```python
from build123d import *

# Parameters (mm, degrees)
SKETCH_1_R      = 2.5
SKETCH_1_R_2    = 3.5
SKETCH_1_R_3    = 3
EXTRUDE_1_DEPTH = 5
FILLET_1_R      = 20
FILLET_2_R      = 20
FILLET_3_R      = 50
FILLET_4_R      = 50
FILLET_5_R      = 50
FILLET_6_R      = 50
FILLET_7_R      = 50
FILLET_8_R      = 50


with BuildPart() as part:
    # 草图1 → 凸台-拉伸1 (new body)
    with BuildSketch(Plane(origin=(4.7625, 0, 0), x_dir=(0, 0, -1), z_dir=(1, 0, 0))):
        Polygon((-227, 0), (-227, -130), (-137, -195), (137, -195), (227, -130), (227, 0), (207, 130), (-207, 130), align=None)
        with Locations((-8, 85)):
            Circle(SKETCH_1_R, mode=Mode.SUBTRACT)
        with Locations((-8, 50)):
            Circle(SKETCH_1_R, mode=Mode.SUBTRACT)
        with Locations(Location((8, 50, 0), (0, 0, 180))):
            Circle(SKETCH_1_R, mode=Mode.SUBTRACT)
        with Locations(Location((8, 85, 0), (0, 0, 180))):
            Circle(SKETCH_1_R, mode=Mode.SUBTRACT)
        with Locations((-100, -175)):
            Circle(SKETCH_1_R_2, mode=Mode.SUBTRACT)
        with Locations((100, -175)):
            Circle(SKETCH_1_R_2, mode=Mode.SUBTRACT)
        with Locations(Location((167, 0, 0), (0, 0, 180))):
            Circle(SKETCH_1_R_2, mode=Mode.SUBTRACT)
        with Locations(Location((87, 0, 0), (0, 0, 180))):
            Circle(SKETCH_1_R_2, mode=Mode.SUBTRACT)
        with Locations(Location((-87, 0, 0), (0, 0, 180))):
            Circle(SKETCH_1_R_2, mode=Mode.SUBTRACT)
        with Locations(Location((-167, 0, 0), (0, 0, 180))):
            Circle(SKETCH_1_R_2, mode=Mode.SUBTRACT)
        with Locations(Location((-215, -50, 0), (0, 0, 180))):
            Circle(SKETCH_1_R_3, mode=Mode.SUBTRACT)
        Polygon((130, -155), (-130, -155), (-175, -120), (-115, -25), (115, -25), (175, -120), align=None, mode=Mode.SUBTRACT)
        Polygon((-144.568690861, -25), (-202, -25), (-202, -85), (-182.463427703, -85), align=None, mode=Mode.SUBTRACT)
        Polygon((182.463427703, -85), (144.568690861, -25), (202, -25), (202, -85), align=None, mode=Mode.SUBTRACT)
        Polygon((-185.552026081, 105), (-50, 105), (-50, 25), (-197.859718389, 25), align=None, mode=Mode.SUBTRACT)
        Polygon((50, 105), (50, 25), (197.859718389, 25), (185.552026081, 105), align=None, mode=Mode.SUBTRACT)
        with BuildLine():
            ThreePointArc((-215, -113.5), (-218, -110.5), (-215, -107.5))
            ThreePointArc((-215, -107.5), (-200.117904907, -105.540735012), (-186.25, -99.796460718))
            ThreePointArc((-186.25, -99.796460718), (-182.151923789, -100.894536929), (-183.25, -104.99261314))
            ThreePointArc((-183.25, -104.99261314), (-198.564990636, -111.336289969), (-215, -113.5))
        make_face(mode=Mode.SUBTRACT)
    extrude(amount=-EXTRUDE_1_DEPTH)

    # 圆角1
    fillet_1_edges = [part.edges().sort_by_distance(p)[0] for p in [
        (2.2625, 130, 207),
    ]]
    fillet(fillet_1_edges, radius=FILLET_1_R)

    # 圆角2
    fillet_2_edges = [part.edges().sort_by_distance(p)[0] for p in [
        (2.2625, 130, -207),
    ]]
    fillet(fillet_2_edges, radius=FILLET_2_R)

    # 圆角3
    fillet_3_edges = [part.edges().sort_by_distance(p)[0] for p in [
        (2.2625, 0, 227),
    ]]
    fillet(fillet_3_edges, radius=FILLET_3_R)

    # 圆角4
    fillet_4_edges = [part.edges().sort_by_distance(p)[0] for p in [
        (2.2625, 0, -227),
    ]]
    fillet(fillet_4_edges, radius=FILLET_4_R)

    # 圆角5
    fillet_5_edges = [part.edges().sort_by_distance(p)[0] for p in [
        (2.2625, -130, 227),
    ]]
    fillet(fillet_5_edges, radius=FILLET_5_R)

    # 圆角6
    fillet_6_edges = [part.edges().sort_by_distance(p)[0] for p in [
        (2.2625, -195, 137),
    ]]
    fillet(fillet_6_edges, radius=FILLET_6_R)

    # 圆角7
    fillet_7_edges = [part.edges().sort_by_distance(p)[0] for p in [
        (2.2625, -195, -137),
    ]]
    fillet(fillet_7_edges, radius=FILLET_7_R)

    # 圆角8
    fillet_8_edges = [part.edges().sort_by_distance(p)[0] for p in [
        (2.2625, -130, -227),
    ]]
    fillet(fillet_8_edges, radius=FILLET_8_R)


solid = part.part
```
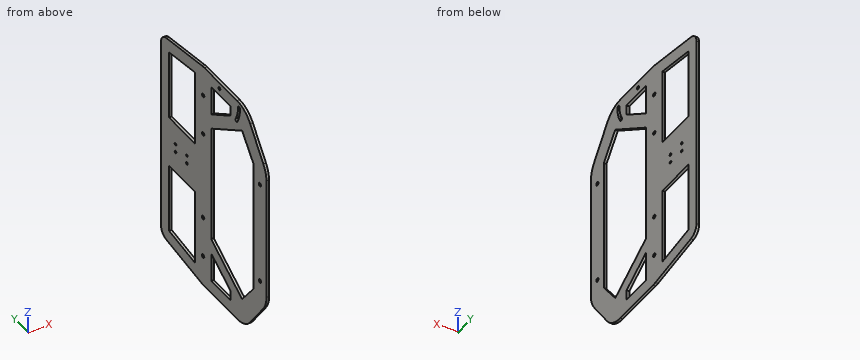
Here's how the part is built. I have some questions about the finished solid (model axes, mm). Coordinates: 2 decimals unless noted, no trailing zeros. Loops run counter-clockwise (first coordinate to the right, second up) from the corner with the lowest first, then second, coordinate; pieces in that order, holes last. Notation, with made-up numbers: M 0.5,6.25 L 43.5,6.25 A28 cw 43.5,41.25 Z; hole C -29,84.25 d8. An arc over 180 degrees is marked long. One line per item, written item: value.
1. Imagine slicing it at D-D (x = 2). State how many separate pieces and enclosed holes the cut face has, and give its area (3 significant figures).
Geometry says:
separate pieces: 1
enclosed holes: 17
area: 72,700 mm2
2. Please list where these lines run through material, in increasing order: probe 1 along Y at (x, z) = (2.65, 8.5); probe 2 along Y at (x, z) = (0.45, -75); probe 3 along Y at (x, z) = (1.85, -8).
Geometry says:
probe 1: y = -195 to -155, -25 to 47.55, 52.45 to 82.55, 87.45 to 130
probe 2: y = -195 to -155, -25 to 25, 105 to 130
probe 3: y = -195 to -155, -25 to 47.5, 52.5 to 82.5, 87.5 to 130
3. Imagine slicing it at B-B (y = -74). List the corners of the cut face in (x, z) for me, and give its area (3 significant figures).
Geometry says:
outline: M -0.24,-227 L 4.76,-227 L 4.76,-202 L -0.24,-202 Z; M -0.24,-175.52 L 4.76,-175.52 L 4.76,-145.95 L -0.24,-145.95 Z; M -0.24,145.95 L 4.76,145.95 L 4.76,175.52 L -0.24,175.52 Z; M -0.24,202 L 4.76,202 L 4.76,227 L -0.24,227 Z
area: 546 mm2
4. Will these pins go through, and if not, where does the flat tip stop? pin 1 Ø11 at (y, z) = (-175, -100) entering from +X; pin 2 Ø2.5 at (x, y) = (2.5, 53.5) entering from -Z.
Geometry says:
pin 1: stops at x = 4.76
pin 2: stops at z = -218.96
5. Imagine slicing it at C-C (y = 59). List the corners of the cut face in (x, z) for me.
Geometry says:
outline: M -0.24,-217.92 L 4.76,-217.92 L 4.76,-192.63 L -0.24,-192.63 Z; M -0.24,-50 L 4.76,-50 L 4.76,50 L -0.24,50 Z; M -0.24,192.63 L 4.76,192.63 L 4.76,217.92 L -0.24,217.92 Z
6. Imagine slicing it at A-A (z = 19.5). List the corners of the cut face in (x, y) for me.
Geometry says:
outline: M -0.24,-195 L 4.76,-195 L 4.76,-155 L -0.24,-155 Z; M -0.24,-25 L 4.76,-25 L 4.76,130 L -0.24,130 Z
